from build123d import *

# Parameters (mm, degrees)
F0_W     = 20
F0_H     = 20
F1_DEPTH = 20
F2_W     = 13
F2_H     = 10
F3_DEPTH = 20
F4_R     = 2
F5_DEPTH = 20
F6_R     = 9.99999
F7_SIZE  = 1


# Not quite as in the source:
# - a fillet or chamfer is up to 0.001 mm smaller than in the source, because OpenCascade refuses the exact size


with BuildPart() as f1:
    # F0 (on Front) → F1 (new body)
    with BuildSketch(Plane.XZ):
        with Locations((10, 10)):
            Rectangle(F0_W, F0_H)
    extrude(amount=-F1_DEPTH)

    # F2 (on face) → F3 (cut, through all)
    with BuildSketch(Plane.YZ.offset(20)):
        with Locations((13.5, 10)):
            Rectangle(F2_W, F2_H)
    extrude(amount=-F3_DEPTH, mode=Mode.SUBTRACT)

    # F4 (on face) → F5 (cut, through all)
    with BuildSketch(Plane.XY.offset(20)):
        with Locations((10, 13.75)):
            Circle(F4_R)
    extrude(amount=-F5_DEPTH, mode=Mode.SUBTRACT)

    # F6 (radius 10 in the source; OpenCascade refuses exactly that, so slightly less here)
    f6_edges = [f1.edges().sort_by_distance(p)[0] for p in [
        (0, 20, 2.5),
        (20, 20, 2.5),
        (20, 20, 17.5),
        (0, 20, 17.5),
    ]]
    fillet(f6_edges, radius=F6_R)

    # F7
    f7_edges = [f1.edges().sort_by_distance(p)[0] for p in [
        (0, 0, 10),
        (10, 0, 0),
        (20, 0, 10),
        (10, 0, 20),
        (10, 7, 15),
        (10, 7, 5),
        (20, 7, 10),
        (0, 7, 10),
        (17.071071, 17.071071, 0),
        (10.00001, 20, 2.5),
        (20, 10.00001, 2.5),
        (17.071071, 17.071071, 5),
        (20, 5.000005, 20),
        (20, 10.00001, 17.5),
        (20, 8.500005, 15),
        (20, 5.000005, 0),
        (20, 8.500005, 5),
        (17.071071, 17.071071, 15),
        (10.00001, 20, 17.5),
        (17.071071, 17.071071, 20),
    ]]
    chamfer(f7_edges, length=F7_SIZE)


solid = f1.part
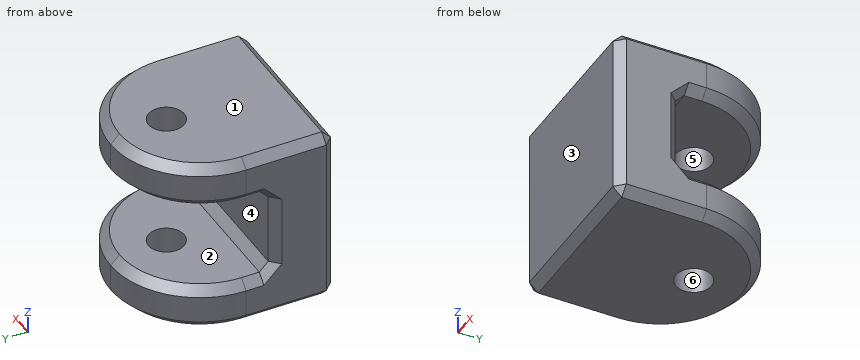
Verification items for the finished model (mm, model axes). Face numbers are marked on the shaded views. A direction names the side the tool comes from. Give positions to 0.01 mm unless a question says otherwise; leave off trailing zeros. Write each loop counter-clockwise with the first axis right and the second up, starting at its lowest first coordinate (ties: lowest second). Pieces come first, ordered by that corner, then holes.
(1) Gauge pin test, flat ends, axial feed: pin 1 (5.5 mm diameter, centred on x = 10, y = 15.5, fed in from +Z); pin 2 (6.5 mm diameter, centred on x = 8.5, z = 9, fed in from +Y); pin 3 (2 mm diameter, centred on x = 2, z = 3.5, fed in from +Y). Record the tip position at first contact, or that the pin passes through.
(2) Cross-section at B-B (z = 9.25). Enter the section's corners in (x, y).
(3) Cross-section at C-C (y = 13.75). State how many separate pieces and enclosed holes the cut face has, plus the area to 3 significant figures.
(4) Access from +Z, -Z, +X, -X, +Y, -Y to the whole of each face (thin tool, end or side, straight path). Record for the marked faces 1 and 2.
(5) Mould release check, pull along Y, two halves, no side actions. Record for the marked faces 3, 4, 5 and 6: +Y half, -Y half, draft (parallel to the pull), parting line (faces both ways), or undercut.
(6) Material ranges on line 1 (Z direction, x = 8, y = 14.75); line 2 (Y direction, x = 10, z = 18.25); line 3 (Y direction, x = 12.25, z = 8.5), recorded low to high.
Worked out:
1. pin 1: stops at z = 20
1. pin 2: stops at y = 7.25
1. pin 3: stops at y = 17.14
2. outline: (0, 1) - (1, 0) - (19, 0) - (20, 1) - (20, 6) - (19, 7) - (1, 7) - (0, 6) - close
3. separate pieces: 4
3. enclosed holes: 0
3. area: 141 mm2
4. face 1: +Z, +X, -X, +Y, -Y
4. face 2: +X, -X, +Y
5. face 3: -Y half
5. face 4: +Y half
5. face 5: undercut
5. face 6: undercut
6. line 1: z = 0 to 5, 15 to 20
6. line 2: y = 0 to 11.75, 15.75 to 20
6. line 3: y = 0 to 7
